from build123d import *

# Parameters (mm, degrees)
SKETCH1_R           = 3
SKETCH1_R_2         = 2.5
BOSS_EXTRUDE1_DEPTH = 300


with BuildPart() as part:
    # Sketch1 → Boss-Extrude1 (new body)
    with BuildSketch(Plane(origin=(0, 0, 0), x_dir=(1, 0, 0), z_dir=(0, 1, 0))):
        with BuildLine():
            Line((-3, -15), (-3, -12.8))
            Line((-3, -12.8), (-5.55, -12.8))
            Line((-5.55, -12.8), (-5.55, -7))
            ThreePointArc((-5.55, -7), (0, -5.16), (5.55, -7))
            Line((5.55, -7), (5.55, -12.8))
            Line((5.55, -12.8), (3, -12.8))
            Line((3, -12.8), (3, -15))
            Line((3, -15), (15, -15))
            Line((15, -15), (15, -3))
            Line((15, -3), (12.8, -3))
            Line((12.8, -3), (12.8, -5.55))
            Line((12.8, -5.55), (7, -5.55))
            ThreePointArc((7, -5.55), (5.16, 0), (7, 5.55))
            Line((7, 5.55), (12.8, 5.55))
            Line((12.8, 5.55), (12.8, 3))
            Line((12.8, 3), (15, 3))
            Line((15, 3), (15, 15))
            Line((15, 15), (3, 15))
            Line((3, 15), (3, 12.8))
            Line((3, 12.8), (5.55, 12.8))
            Line((5.55, 12.8), (5.55, 7))
            ThreePointArc((5.55, 7), (0, 5.16), (-5.55, 7))
            Line((-5.55, 7), (-5.55, 12.8))
            Line((-5.55, 12.8), (-3, 12.8))
            Line((-3, 12.8), (-3, 15))
            Line((-3, 15), (-15, 15))
            Line((-15, 15), (-15, 3))
            Line((-15, 3), (-12.8, 3))
            Line((-12.8, 3), (-12.8, 5.55))
            Line((-12.8, 5.55), (-7, 5.55))
            ThreePointArc((-7, 5.55), (-5.16, 0), (-7, -5.55))
            Line((-7, -5.55), (-12.8, -5.55))
            Line((-12.8, -5.55), (-12.8, -3))
            Line((-12.8, -3), (-15, -3))
            Line((-15, -3), (-15, -15))
            Line((-15, -15), (-3, -15))
        make_face()
        with Locations(Location((-10, 10, 0), (0, 0, 270))):
            Circle(SKETCH1_R, mode=Mode.SUBTRACT)
        with Locations(Location((10, 10, 0), (0, 0, 270))):
            Circle(SKETCH1_R, mode=Mode.SUBTRACT)
        with Locations(Location((-10, -10, 0), (0, 0, 270))):
            Circle(SKETCH1_R, mode=Mode.SUBTRACT)
        with Locations(Location((10, -10, 0), (0, 0, 270))):
            Circle(SKETCH1_R, mode=Mode.SUBTRACT)
        with Locations(Location((0, 0, 0), (0, 0, 270))):
            Circle(SKETCH1_R_2, mode=Mode.SUBTRACT)
    extrude(amount=BOSS_EXTRUDE1_DEPTH)


solid = part.part
Could you check a few things on this model? Use its own coordinates, in mm. A direction names the side the tool comes from. Round coordinates to 2 decimals unless told otherwise and drop trailing zeros. Order: outer loops, then holes, each group sorted by start corner. A loop starts at its lowest first (then second) coordinate and runs counter-clockwise, first axis right, second up. Notation, with made-up numbers: M 23,23.25 L 49,23.25 A11 cw 49,43.25 Z; hole C 86,2 d9. An arc over 180 degrees is marked long. One line per item, written item: value.
(1) Which directions (+Z, -Z, +X, -X, +Y, -Y) give clear straight access to the entire face, cutting with the end or side of a thin tool? Please do faces 1 (the flat face through (-9, 148, 15)), 2 (the flat face through (5.55, 148, -10)).
Ans:
face 1: +Z, +X, -X, +Y, -Y
face 2: +Y, -Y
(2) I'm going to push a flat-ended pin straight in: P1, Ø1, axis at x = 1, y = 77, coming from the +Z side. Where does the tip first touch, or does it pass through?
Ans:
P1: stops at z = 5.28
(3) I need wall thicknesses on line 1 along X through (y, z) = (216, -9.5); line 2 along X through (y, z) = (205.5, 0); line 3 along Z through (x, y) = (10.75, 159). Which ranges of each line are inside material? Lowest first, please. Write a range as from..to.
Ans:
line 1: x = -15..-12.96, -7.04..-5.55, 5.55..7.04, 12.96..15
line 2: x = -5.16..-2.5, 2.5..5.16
line 3: z = -15..-12.9, -7.1..-5.55, 5.55..7.1, 12.9..15
(4) If we mould it in two halves opening along X, with no side actions, what happens to faces 3 (the flat face through (-9, 148, -15)), 4 (the cylindrical face through (10, 148, -13)), 5 (the flat face through (-15, 148, 9)), 6 (the flat face through (-5.55, 148, -10))? For each: released by +X, released by -X, zero draft, split by the parting line, or undercut.
Ans:
face 3: zero draft
face 4: undercut
face 5: released by -X
face 6: undercut
(5) Imagine slicing it at B-B (z = 10). Write out the boundary of the cut face in (x, y), and give its area (3 significant figures).
Ans:
outline: M -15,0 L -13,0 L -13,300 L -15,300 Z; M -7,0 L -5.55,0 L -5.55,300 L -7,300 Z; M 5.55,0 L 7,0 L 7,300 L 5.55,300 Z; M 13,0 L 15,0 L 15,300 L 13,300 Z
area: 2,070 mm^2
(6) Imagine slicing it at C-C (y = 246.5). Count the separate pieces of the cut face and the enclosed holes in it, and give its area (3 significant figures).
Ans:
separate pieces: 1
enclosed holes: 5
area: 401 mm^2
(7) Imagine slicing it at A-A (x = 0). Write out the boundary of the cut face in (y, z), and give its area (3 significant figures).
Ans:
outline: M 0,-5.16 L 300,-5.16 L 300,-2.5 L 0,-2.5 Z; M 0,2.5 L 300,2.5 L 300,5.16 L 0,5.16 Z
area: 1,600 mm^2
